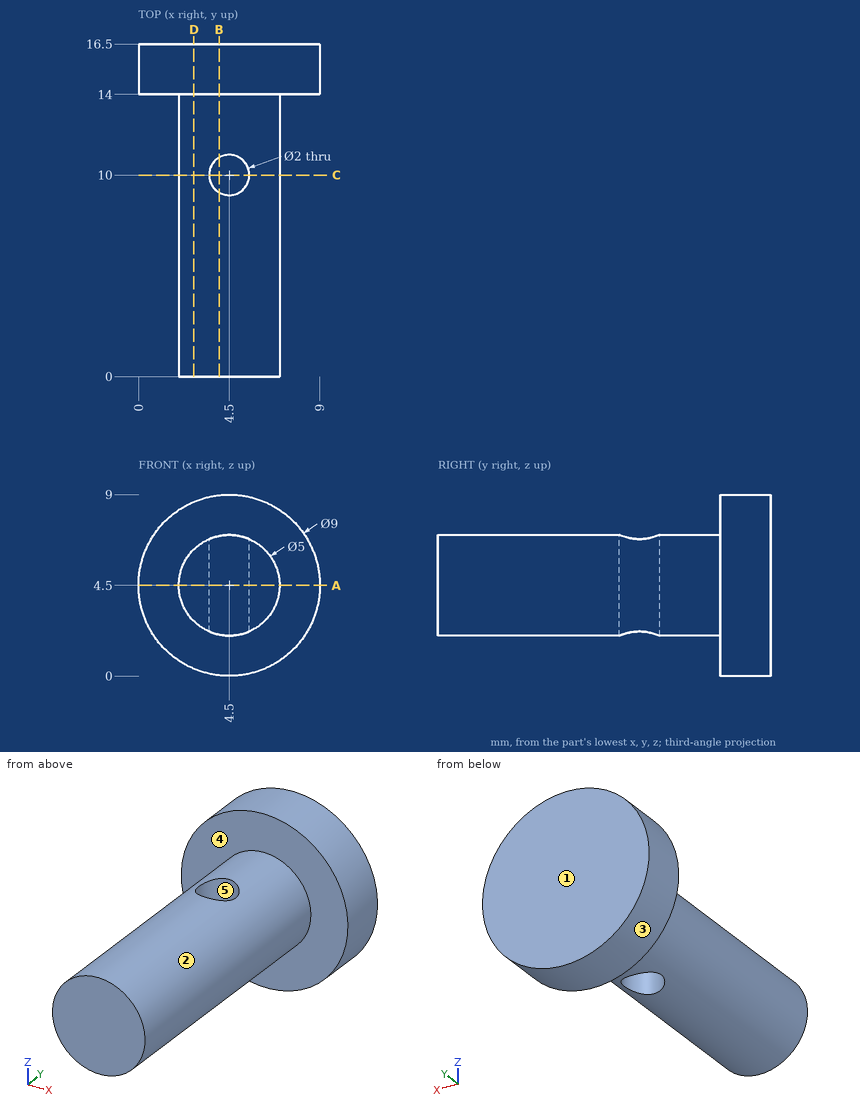
Geometry check sheet. Reference: drawing and pictorial views, mm from the part's lowest x, y, z. A direction names the side the tool comes from. Give positions to 0.01 mm unless a question says otherwise; leave off trailing zeros. Order: outer loops, then holes, each group sorted by start corner. A loop starts at its lowest first (then second) coordinate and runs counter-clockwise, first axis right, second up. Notation, with made-up numbers: M 48,6.25 L 100,6.25 A10 cw 100,13.25 Z; hole C 73.5,13.5 d4. An arc over 180 degrees is marked long. Answer in a Markdown table with one row per item.
1) Cross-section at A-A, the plane z = 4.5. Enter the section's corners in (x, y), plus the area to 3 significant figures.
Filled sheet:
| item | result |
|---|---|
| outline | M 0,14 L 2,14 L 2,0 L 7,0 L 7,14 L 9,14 L 9,16.5 L 0,16.5 Z; hole C 4.5,10 d2 |
| area | 89.4 mm2 |
2) Cross-section at B-B, the plane x = 4. Enter the section's corners in (y, z), plus the area to 3 significant figures.
Filled sheet:
| item | result |
|---|---|
| outline | M 0,2.05 L 9.13,2.05 L 9.13,6.95 L 0,6.95 Z; M 10.87,2.05 L 14,2.05 L 14,0.03 L 16.5,0.03 L 16.5,8.97 L 14,8.97 L 14,6.95 L 10.87,6.95 Z |
| area | 82.5 mm2 |
3) Cross-section at D-D, the plane x = 2.75. Enter the section's corners in (y, z).
Filled sheet:
| item | result |
|---|---|
| outline | M 0,2.71 L 14,2.71 L 14,0.35 L 16.5,0.35 L 16.5,8.65 L 14,8.65 L 14,6.29 L 0,6.29 Z |
4) Release check for a two-part mould opening along X. For the marked faces 3, 4 and 5 record: +X half, -X half, draft (parallel to the pull), parting line (faces both ways), or undercut.
Filled sheet:
| item | result |
|---|---|
| face 3 | parting line |
| face 4 | draft |
| face 5 | undercut |
5) Gauge pin test, flat ends, axial feed: P1, Ø5, axis at y = 7, z = 4, coming from the -X side; P2, Ø1.6, axis at x = 4.5, y = 10, coming from the -Z side; P3, Ø1, axis at y = 8, z = 5.5, coming from the -X side; P4, Ø3, axis at x = 7, z = 8, coming from the -Y side. Record the tip position at first contact, or that the pin passes through.
Filled sheet:
| item | result |
|---|---|
| P1 | stops at x = 2 |
| P2 | passes through |
| P3 | stops at x = 2.05 |
| P4 | stops at y = 14 |
6) Access from +Z, -Z, +X, -X, +Y, -Y to the whole of each face (thin tool, end or side, straight path). Record for the marked faces 1 and 2.
Filled sheet:
| item | result |
|---|---|
| face 1 | +Z, -Z, +X, -X, +Y |
| face 2 | -Y |
7) Cross-section at C-C, the plane y = 10. Enter the section's corners in (x, z), plus the area to 3 significant figures.
Filled sheet:
| item | result |
|---|---|
| outline | M 3.5,2.21 L 3.5,6.79 A2.5 ccw Z; M 5.5,2.21 A2.5 ccw 5.5,6.79 Z |
| area | 9.91 mm2 |
8) Thickness scan on L1, parallel to X at y = 10, z = 4.35; L2, parallel to X at y = 10, z = 3.45; L3, parallel to Y at x = 2.25, z = 2. Record the ranges inside material, lowest first. Write a range as [from, to].
Filled sheet:
| item | result |
|---|---|
| L1 | x = [2, 3.5], [5.5, 7] |
| L2 | x = [2.23, 3.5], [5.5, 6.77] |
| L3 | y = [14, 16.5] |
